from build123d import *

# Parameters (mm, degrees)
SKETCH_1_R      = 2.5
SKETCH_1_W      = 350
SKETCH_1_H      = 223.275
EXTRUDE_1_DEPTH = 2


with BuildPart() as part:
    # 草图1 → 凸台-拉伸1 (new body)
    with BuildSketch(Plane.XY):
        Polygon((70, 580), (650, 580), (650, 0), (535, 0), (535, 150.575), (185, 150.575), (185, 0), (70, 0), align=None)
        with Locations((175.620271067, 285.3)):
            Circle(SKETCH_1_R, mode=Mode.SUBTRACT)
        with Locations((175.620271067, 239.279728933)):
            Circle(SKETCH_1_R, mode=Mode.SUBTRACT)
        with Locations((169.3, 262.3)):
            Circle(SKETCH_1_R, mode=Mode.SUBTRACT)
        with Locations((169.3, 303.1)):
            Circle(SKETCH_1_R, mode=Mode.SUBTRACT)
        with Locations((549.420271067, 285.3)):
            Circle(SKETCH_1_R, mode=Mode.SUBTRACT)
        with Locations((549.420271067, 239.279728933)):
            Circle(SKETCH_1_R, mode=Mode.SUBTRACT)
        with Locations((543.1, 262.3)):
            Circle(SKETCH_1_R, mode=Mode.SUBTRACT)
        with Locations((543.1, 303.1)):
            Circle(SKETCH_1_R, mode=Mode.SUBTRACT)
        with Locations((360, 313.3625)):
            Rectangle(SKETCH_1_W, SKETCH_1_H, mode=Mode.SUBTRACT)
    extrude(amount=EXTRUDE_1_DEPTH)


solid = part.part
Source: CAD feature listing. Evaluate the final solid. Frame: model axes, mm. Coordinates: 2 decimals unless noted, no trailing zeros. Order: outer loops, then holes, each group sorted by start corner. A loop starts at its lowest first (then second) coordinate and runs counter-clockwise, first axis right, second up. Notation, with made-up numbers: M 88.25,-4.75 L 128.25,-4.75 A27 cw 128.25,24.25 Z; hole C 29.5,57 d11. An arc over 180 degrees is marked long. Write each question's results on one line, items separated by ' | '. Start each with the question number.
1. Section C-C, the plane z = 1.6. State how many separate pieces and enclosed holes the cut face has, then the cut area to 3 significant figures.
2. Section A-A, the plane y = 39.5. Return the cut outline in (x, z).
3. Pin query (flat end, axial travel): pin 1 (1 mm diameter, centred on x = 431, z = 0.5, fed in from -Y) (3 decimals). Return the tip coordinate at first contact, or that it passes through.
4. Material intervals for L1, parallel to Y at x = 169.3, z = 1.3; L2, parallel to X at y = 262.3, z = 1.45; L3, parallel to Y at x = 210.5, z = 1.25 (3 decimals), sorted ascending.
5. Section B-B, the plane x = 327. Return the cut outline in (y, z) (3 decimals), then the cut area to 3 significant figures.
Solution:
1) separate pieces: 1 | enclosed holes: 9 | area: 205,000 mm²
2) outline: M 70,0 L 185,0 L 185,2 L 70,2 Z; M 535,0 L 650,0 L 650,2 L 535,2 Z
3) pin 1: y = 150.575
4) L1: 0 to 259.8, 264.8 to 300.6, 305.6 to 580 | L2: 70 to 166.8, 171.8 to 185, 535 to 540.6, 545.6 to 650 | L3: 150.575 to 201.725, 425 to 580
5) outline: M 150.575,0 L 201.725,0 L 201.725,2 L 150.575,2 Z; M 425,0 L 580,0 L 580,2 L 425,2 Z | area: 412 mm²
